Could you check a few things on this drawing? It's one solid part, dimensions in mm from its lowest x, y, z. Give positions to 0.01 mm unless a question says otherwise; leave off trailing zeros. Order: outer loops, then holes, each group sorted by start corner. A loop starts at its lowest first (then second) coordinate and runs counter-clockwise, first axis right, second up.
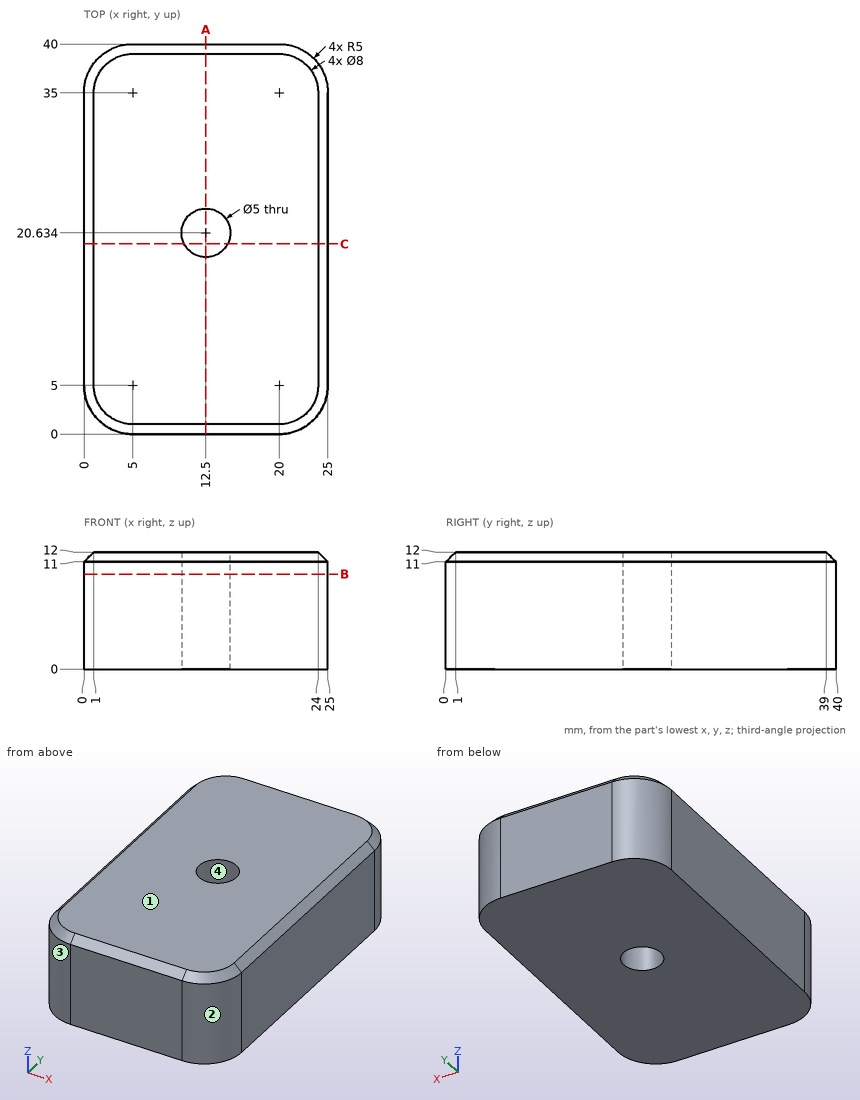
Q1. If we section it at A-A on x = 12.5: List the corners of the cut face in (y, z) for me.
Filled sheet:
outline: (0, 0) - (18.13, 0) - (18.13, 12) - (1, 12) - (0, 11) - close; (23.13, 0) - (40, 0) - (40, 11) - (39, 12) - (23.13, 12) - close
Q2. If we section it at C-C on y = 19.5: List the corners of the cut face in (x, z) for me.
Filled sheet:
outline: (0, 0) - (10.27, 0) - (10.27, 12) - (1, 12) - (0, 11) - close; (14.73, 0) - (25, 0) - (25, 11) - (24, 12) - (14.73, 12) - close
Q3. If we section it at B-B on z = 9.75: List the corners of the cut face in (x, y) for me, plus the area to 3 significant figures.
Filled sheet:
outline: (0, 5) arc R5 ccw to (5, 0) - (20, 0) arc R5 ccw to (25, 5) - (25, 35) arc R5 ccw to (20, 40) - (5, 40) arc R5 ccw to (0, 35) - close; hole circle Ø5 at (12.5, 20.63)
area: 959 mm2
Q4. Thinking about a two-plate mould opening in X: for the marked faces 1, 2, 3 and 4, which applies, released by +X, released by -X, zero draft, split by the parting line, or undercut?
Filled sheet:
face 1: zero draft
face 2: released by +X
face 3: released by -X
face 4: undercut
Q5. I need wall thicknesses on L1, parallel to Y at x = 12.5, z = 7.25; L2, parallel to Y at x = 13.25, z = 2.25; L3, parallel to X at y = 20, z = 2.25. Which ranges of each line are inside material? Lowest first, please.
Filled sheet:
L1: y = 0 to 18.13, 23.13 to 40
L2: y = 0 to 18.25, 23.02 to 40
L3: x = 0 to 10.08, 14.92 to 25
